Verification items for the finished model (mm, model axes). A direction names the side the tool comes from. Round coordinates to 2 decimals unless told otherwise and drop trailing zeros. Order: outer loops, then holes, each group sorted by start corner. A loop starts at its lowest first (then second) coordinate and runs counter-clockwise, first axis right, second up. Notation, with made-up numbers: M -9,13.5 L 47,13.5 A20 ccw 47,35.5 Z; hole C -7,26 d6. An arc over 180 degrees is marked long. Use one line per item in the form item = value. Start each with the question number.
Item 1: Release check for a two-part mould opening along Y. For faces 1 (the cylindrical face through (7.709, 34.714, 14.752)), 2 (the conical face through (40.56, 7.79, 8.23)), 3 (the flat face through (-31.64, -26.55, 3.88)), 4 (the flat face through (-7.17, 40.67, 3.88)) record: +Y half, -Y half, draft (parallel to the pull), parting line (faces both ways), or undercut.
Item 2: Thickness scan on probe 1 along X at (y, z) = (0, 10.8); probe 2 along Y at (x, z) = (0, 14.75); probe 3 along Y at (x, z) = (-31.5, 6.25). Record the ranges inside material, lowest first. Write a range as [from, to].
Item 3: Tool access check on faces 5 (the flat face through (-41, 0, 4)), 6 (the flat face through (20.65, 35.77, 3.88)), 7 (the flat face through (38.811, -14.126, 3.88)). Record the directions out of +Z, -Z, +X, -X, +Y, -Y that give a thin tool (end or side, any length) a straight path to the whole face; none if there is none.
Item 4: Go/stop test with flat-tipped pins: pin 1 Ø4 at (y, z) = (-25, 9) entering from -X; pin 2 Ø4 at (x, z) = (1, 13.5) entering from -Y; pin 3 Ø3 at (y, z) = (16, 12) entering from +X; pin 4 Ø4 at (x, y) = (-32.5, 30.5) entering from -Z. Record where each tip stops, or that it passes through.
Item 5: Cross-section at A-A on x = 0. Enter the section's corners in (y, z) (3 decimals).
from build123d import *

# Parameters (mm, degrees)
F3_DEPTH        = 25.4
F3_COPIES_COUNT = 9


# Not quite as in the source:
# - a pattern or mirror of a feature is missing from the dataset's text; its kind, count and spacing are read off the source's solid


with BuildPart() as f1:
    # F0 (on Front) → F1 (revolve)
    with BuildSketch(Plane.XZ):
        with BuildLine():
            Line((-43.18, 15.875), (-43.18, 0))
            Line((-43.18, 0), (-35.56, 0))
            Line((-35.56, 0), (-34.29, 7.747))
            Line((-34.29, 7.747), (-34.29, 11.8019743879))
            ThreePointArc((-34.29, 11.8019743879), (-34.3383364969, 12.0449783674), (-34.4759871939, 12.2509871939))
            Line((-34.4759871939, 12.2509871939), (-35.3740128061, 13.1490128061))
            ThreePointArc((-35.3740128061, 13.1490128061), (-35.5116635031, 13.3550216326), (-35.56, 13.5980256121))
            Line((-35.56, 13.5980256121), (-35.56, 15.875))
            Line((-35.56, 15.875), (-43.18, 15.875))
        make_face()
    revolve(axis=Axis((0, 0, 20.137766609), (0, 0, 1)))

    # F2 (on face) → F3 (cut)
    with BuildSketch(Plane(origin=(0, 0, 0), x_dir=(1, 0, 0), z_dir=(0, 0, -1))):
        with BuildLine():
            Line((-49.9110633764, 0), (-39.37, 0))
            ThreePointArc((-39.37, 0), (-38.6466622123, 7.512150148), (-36.5032283543, 14.7482615828))
            Line((-36.5032283543, 14.7482615828), (-46.2767321268, 18.6970134252))
            ThreePointArc((-46.2767321268, 18.6970134252), (-48.994056565, 9.523479861), (-49.9110633764, 0))
        make_face()
    f3 = extrude(amount=-F3_DEPTH, mode=Mode.SUBTRACT)

    # F3_copies: F3 ×9 about axis
    f3_copies_axis = Axis((0, 0, 0), (0, 0, 1))
    for i in range(1, F3_COPIES_COUNT):
        add(f3.rotate(f3_copies_axis, i * 360 / F3_COPIES_COUNT), mode=Mode.SUBTRACT)

    # F5 (on Right) → F6 (revolve, cut)
    with BuildSketch(Plane.YZ):
        Polygon((39.37, 15.875), (39.37, 10.16), (43.18, 6.35), (43.18, 15.875), align=None)
    revolve(axis=Axis((0, 0, 20.137766609), (0, 0, 1)), mode=Mode.SUBTRACT)


solid = f1.part
Output values:
q1.face_1 = undercut
q1.face_2 = +Y half
q1.face_3 = -Y half
q1.face_4 = undercut
q2.probe_1 = [-39.37, -34.29], [34.29, 39.37]
q2.probe_2 = [-39.37, -35.56], [35.56, 39.37]
q2.probe_3 = [-26.43, -14.16], [14.16, 23.62], [26.43, 29.53]
q3.face_5 = +Z, -Z, -X
q3.face_6 = +Z, -Z, +Y
q3.face_7 = +Z, -Z, +X
q4.pin_1 = -34.79
q4.pin_2 = -39.37
q4.pin_3 = 36.6
q4.pin_4 = 0
q5.outline = M -39.37,0 L -35.56,0 L -34.29,7.747 L -34.29,11.802 A0.635 ccw -34.476,12.251 L -35.374,13.149 A0.635 cw -35.56,13.598 L -35.56,15.875 L -39.37,15.875 Z; M 34.29,7.747 L 35.56,0 L 43.18,0 L 43.18,6.35 L 39.37,10.16 L 39.37,15.875 L 35.56,15.875 L 35.56,13.598 A0.635 cw 35.374,13.149 L 34.476,12.251 A0.635 ccw 34.29,11.802 Z
